```python
from build123d import *

# Parameters (mm, degrees)
SKETCH_2_W                 = 48
SKETCH_2_H                 = 75
EXTRUDE_1_DEPTH            = 10
EXTRUDE_2_DEPTH            = 55
EXTRUDE_2_DEPTH_BACK       = 10
SKETCH_5_W                 = 10
SKETCH_5_H                 = 10
EXTRUDE_2_2_DEPTH          = 55
EXTRUDE_2_2_DEPTH_BACK     = 10
SKETCH_5_H_2               = 20
EXTRUDE_2_3_DEPTH          = 55
EXTRUDE_2_3_DEPTH_BACK     = 10
EXTRUDE_2_4_DEPTH          = 55
EXTRUDE_2_4_DEPTH_BACK     = 10
EXTRUDE_3_DEPTH            = 5
SKETCH_7_R                 = 2.5
CUT_EXTRUDE_1_DEPTH        = 10
FILLET_1_R                 = 10
SKETCH_8_R                 = 1.5
CUT_EXTRUDE_2_DEPTH        = 121.205647632
PATTERN_LINEAR_1_COUNT     = 2
PATTERN_LINEAR_1_PITCH     = 15
PATTERN_LINEAR_1_COL_COUNT = 2
PATTERN_LINEAR_1_COL_PITCH = 15
SKETCH_10_R                = 1.5
CUT_EXTRUDE_4_DEPTH        = 10
SKETCH_11_R                = 1.5
CUT_EXTRUDE_5_DEPTH        = 5
FILLET_9_R                 = 2.5
EXTRUDE_5_DEPTH            = 5
FILLET_10_R                = 5
FILLET_11_R                = 5
SKETCH_14_R                = 1.5
CUT_EXTRUDE_6_DEPTH        = 5
SKETCH_15_W                = 5
SKETCH_15_H                = 2
CUT_EXTRUDE_7_DEPTH        = 55
SKETCH_17_R                = 1.5
CUT_EXTRUDE_10_DEPTH       = 118.336631714


with BuildPart() as part:
    # Sketch 2 → Extrude 1 (new body)
    with BuildSketch(Plane(origin=(0, 0, 0), x_dir=(0, 0, -1), z_dir=(1, 0, 0))):
        with Locations((22.061440678, -32.335805085)):
            Rectangle(SKETCH_2_W, SKETCH_2_H)
    extrude(amount=EXTRUDE_1_DEPTH)



with BuildPart() as body_2:
    # Sketch 5 → Extrude 2 (new, two sides: drawn at the far end of the back side and taken through both)
    with BuildSketch(Plane(origin=(10, 0, 0), x_dir=(0, 0, -1), z_dir=(1, 0, 0)).offset(-EXTRUDE_2_DEPTH_BACK)):
        with Locations((51.061440678, 0.164194915)):
            Rectangle(SKETCH_5_W, SKETCH_5_H)
    extrude(amount=EXTRUDE_2_DEPTH + EXTRUDE_2_DEPTH_BACK)


with BuildPart() as body_3:
    # Sketch 5 → Extrude 2 2 (new, two sides: drawn at the far end of the back side and taken through both)
    with BuildSketch(Plane(origin=(10, 0, 0), x_dir=(0, 0, -1), z_dir=(1, 0, 0)).offset(-EXTRUDE_2_2_DEPTH_BACK)):
        with Locations((51.061440678, -59.835805085)):
            Rectangle(SKETCH_5_W, SKETCH_5_H_2)
    extrude(amount=EXTRUDE_2_2_DEPTH + EXTRUDE_2_2_DEPTH_BACK)


with BuildPart() as body_4:
    # Sketch 5 → Extrude 2 3 (new, two sides: drawn at the far end of the back side and taken through both)
    with BuildSketch(Plane(origin=(10, 0, 0), x_dir=(0, 0, -1), z_dir=(1, 0, 0)).offset(-EXTRUDE_2_3_DEPTH_BACK)):
        with Locations((-6.938559322, -59.835805085)):
            Rectangle(SKETCH_5_W, SKETCH_5_H_2)
    extrude(amount=EXTRUDE_2_3_DEPTH + EXTRUDE_2_3_DEPTH_BACK)


with BuildPart() as body_5:
    # Sketch 5 → Extrude 2 4 (new, two sides: drawn at the far end of the back side and taken through both)
    with BuildSketch(Plane(origin=(10, 0, 0), x_dir=(0, 0, -1), z_dir=(1, 0, 0)).offset(-EXTRUDE_2_4_DEPTH_BACK)):
        with Locations((-6.938559322, 0.164194915)):
            Rectangle(SKETCH_5_W, SKETCH_5_H)
    extrude(amount=EXTRUDE_2_4_DEPTH + EXTRUDE_2_4_DEPTH_BACK)


with BuildPart() as part_1:
    add(part.part)

    add(body_3.part)  # Extrude 3 merges body 3

    add(body_4.part)  # Extrude 3 merges body 4
    # Sketch 6 → Extrude 3 (add)
    with BuildSketch(Plane.XZ.offset(69.835805085)):
        Polygon((65, 1.938559322), (65, 11.938559322), (0, 11.938559322), (0, 1.938559322), (0, -46.061440678), (0, -56.061440678), (65, -56.061440678), (65, -46.061440678), align=None)
    extrude(amount=EXTRUDE_3_DEPTH)

    # Sketch 7 → Cut-Extrude 1 (cut)
    with BuildSketch(Plane.ZY):
        with Locations((-22.061440678, -22.335805085)):
            Circle(SKETCH_7_R)
    extrude(amount=-CUT_EXTRUDE_1_DEPTH, mode=Mode.SUBTRACT)

    # Fillet 1
    fillet_1_edges = [part_1.edges().sort_by_distance(p)[0] for p in [
        (5, -49.835805085, -46.061440678),
        (5, -49.835805085, 1.938559322),
    ]]
    fillet(fillet_1_edges, radius=FILLET_1_R - 0.0001)  # a hair under: the kernel refuses the full size

    # Sketch 8 → Cut-Extrude 2 (cut, through all)
    with BuildSketch(Plane(origin=(0, 0, -56.061440678), x_dir=(-1, 0, 0), z_dir=(0, 0, -1))):
        with Locations((-32.5, -56.085805085)):
            Circle(SKETCH_8_R)
    cut_extrude_2 = extrude(amount=-CUT_EXTRUDE_2_DEPTH, mode=Mode.SUBTRACT)

    # Pattern Linear 1: Cut-Extrude 2 ×2
    with Locations(*[(i * PATTERN_LINEAR_1_PITCH, 0, 0) for i in range(1, PATTERN_LINEAR_1_COUNT)]):
        add(cut_extrude_2, mode=Mode.SUBTRACT)

    # Pattern Linear 1 col: Cut-Extrude 2 ×2
    with Locations(*[(-i * PATTERN_LINEAR_1_COL_PITCH, 0, 0) for i in range(1, PATTERN_LINEAR_1_COL_COUNT)]):
        add(cut_extrude_2, mode=Mode.SUBTRACT)

    # Sketch 10 → Cut-Extrude 4 (cut)
    with BuildSketch(Plane(origin=(0, -69.835805085, 0), x_dir=(1, 0, 0), z_dir=(0, 1, 0))):
        with Locations(Location((15, 2.632869249, 0), (0, 0, 270))):
            Circle(SKETCH_10_R)
        with Locations(Location((15, 41.490012107, 0), (0, 0, 270))):
            Circle(SKETCH_10_R)
    extrude(amount=-CUT_EXTRUDE_4_DEPTH, mode=Mode.SUBTRACT)

    # Sketch 11 → Cut-Extrude 5 (cut)
    with BuildSketch(Plane(origin=(65, 0, 0), x_dir=(0, 0, -1), z_dir=(1, 0, 0))):
        with Locations((51.061440678, -69.835805085)):
            Circle(SKETCH_11_R)
        with Locations((-6.938559322, -69.835805085)):
            Circle(SKETCH_11_R)
    extrude(amount=-CUT_EXTRUDE_5_DEPTH, mode=Mode.SUBTRACT)

    # Fillet 9
    fillet_9_edges = [part_1.edges().sort_by_distance(p)[0] for p in [
        (0, -62.335805085, -56.061440678),
        (0, -62.335805085, 11.938559322),
    ]]
    fillet(fillet_9_edges, radius=FILLET_9_R)


    add(body_2.part)  # Extrude 5 merges body 2

    add(body_5.part)  # Extrude 5 merges body 5
    # Sketch 13 → Extrude 5 (add)
    with BuildSketch(Plane(origin=(0, 5.164194915, 0), x_dir=(1, 0, 0), z_dir=(0, 1, 0))):
        Polygon((0, -11.938559322), (65, -11.938559322), (65, -1.938559322), (10, -1.938559322), (10, 46.061440678), (65, 46.061440678), (65, 56.061440678), (0, 56.061440678), (0, 46.061440678), (0, -1.938559322), align=None)
    extrude(amount=EXTRUDE_5_DEPTH)

    # Fillet 10
    fillet_10_edges = [part_1.edges().sort_by_distance(p)[0] for p in [
        (32.5, 10.164194915, 11.938559322),
        (32.5, -4.835805085, 11.938559322),
    ]]
    fillet(fillet_10_edges, radius=FILLET_10_R)

    # Fillet 11
    fillet_11_edges = [part_1.edges().sort_by_distance(p)[0] for p in [
        (32.5, 10.164194915, -56.061440678),
        (32.5, -4.835805085, -56.061440678),
    ]]
    fillet(fillet_11_edges, radius=FILLET_11_R)

    # Sketch 14 → Cut-Extrude 6 (cut)
    with BuildSketch(Plane(origin=(65, 0, 0), x_dir=(0, 0, -1), z_dir=(1, 0, 0))):
        with Locations((-6.938559322, 2.664194915)):
            Circle(SKETCH_14_R)
        with Locations((51.061440678, 2.664194915)):
            Circle(SKETCH_14_R)
    extrude(amount=-CUT_EXTRUDE_6_DEPTH, mode=Mode.SUBTRACT)

    # Sketch 15 → Cut-Extrude 7 (cut)
    with BuildSketch(Plane(origin=(65, 0, 0), x_dir=(0, 0, -1), z_dir=(1, 0, 0))):
        with Locations((22.061440678, -70.835805085)):
            Rectangle(SKETCH_15_W, SKETCH_15_H)
    extrude(amount=-CUT_EXTRUDE_7_DEPTH, mode=Mode.SUBTRACT)

    # Sketch 17 → Cut-Extrude 10 (cut, through all)
    with BuildSketch(Plane(origin=(0, -69.835805085, 0), x_dir=(1, 0, 0), z_dir=(0, 1, 0))):
        with Locations(Location((60.5, 22.061440678, 0), (0, 0, 270))):
            Circle(SKETCH_17_R)
        with Locations(Location((46.5, 22.061440678, 0), (0, 0, 270))):
            Circle(SKETCH_17_R)
        with Locations(Location((53.5, 29.061440678, 0), (0, 0, 270))):
            Circle(SKETCH_17_R)
        with Locations(Location((53.5, 22.061440678, 0), (0, 0, 270))):
            Circle(SKETCH_17_R)
        with Locations(Location((53.5, 15.061440678, 0), (0, 0, 270))):
            Circle(SKETCH_17_R)
        with Locations(Location((32.5, 15.061440678, 0), (0, 0, 270))):
            Circle(SKETCH_17_R)
        with Locations(Location((39.5, 22.061440678, 0), (0, 0, 270))):
            Circle(SKETCH_17_R)
        with Locations(Location((25.5, 22.061440678, 0), (0, 0, 270))):
            Circle(SKETCH_17_R)
        with Locations(Location((32.5, 22.061440678, 0), (0, 0, 270))):
            Circle(SKETCH_17_R)
        with Locations(Location((32.5, 29.061440678, 0), (0, 0, 270))):
            Circle(SKETCH_17_R)
    extrude(amount=-CUT_EXTRUDE_10_DEPTH, mode=Mode.SUBTRACT)


solid = part_1.part
```
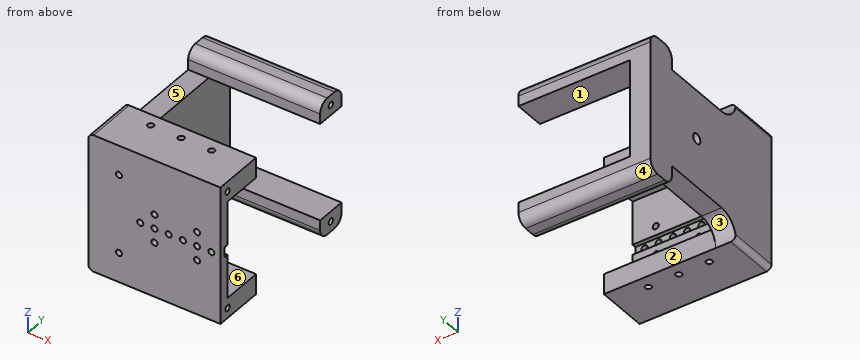
Input: part model. Units: mm. Frame: model coordinates. Face numbers are marked on the shaded views. A direction names the side the tool comes from. Give positions to 0.01 mm unless a question says otherwise; leave off trailing zeros. Order: outer loops, then holes, each group sorted by start corner. A loop starts at its lowest first (then second) coordinate and runs counter-clockwise, first axis right, second up. Notation, with made-up numbers: (36.25, 62) -> (55.25, 62) arc R27 ccw to (55.25, 79) -> close; hole circle Ø3 at (-13.75, 76.5). An arc over 180 degrees is marked (long way). Write each question's results on one line, items separated by ' | '. Start each with the question number.
Item 1: Set-up query: the marked faces 1, 2 and 3. Return all of +Z, -Z, +X, -X, +Y, -Y with unobstructed straight access to the full face (end or side cutting, diameter ignored); none if empty.
Item 2: Cut plane A-A on x = 25.5. Return the cut outline in (y, z).
Item 3: Cut plane C-C on x = 36. Return the cut outline in (y, z), then the cut area to 3 significant figures.
Item 4: Line query: line 1 (Y direction, x = 47.5, z = 4); line 2 (Y direction, x = 29, z = -48); line 3 (Z direction, x = 21, y = -63). Output: solid intervals per line, ascending.
Item 5: Cut plane D-D on z = -22. Give the number of separate pieces and of enclosed holes in the cut face, then the cut area to 3 significant figures.
Item 6: Mould query, pull axis Z, two halves, no side actions, for the marked faces 4, 5 and 6. Classes: pulls with the +Z half, pulls with the -Z half, needs draft (parallel to the pull), parting line crosses it, or undercut.
Item 7: Cut plane B-B on z = -15. Return the cut outline in (x, y).
Item 8: Contact query for flat-ended pins moving along their axis: P1, Ø5, axis at x = 55, y = -4, coming from the +Z side; P2, Ø8, axis at y = -36.5, z = -45.5, coming from the +X side; P3, Ø6, axis at x = 48.5, z = -17, coming from the +Y side. Output: stop coordinate, or through.
Established:
1) face 1: +X, +Y | face 2: +Z, -Z, +X | face 3: -Z, +X, -X
2) outline: (-74.84, -56.06) -> (-49.84, -56.06) -> (-49.84, -46.06) -> (-69.84, -46.06) -> (-69.84, -24.56) -> (-71.84, -24.56) -> (-71.84, -23.56) -> (-74.84, -23.56) -> close; (-74.84, -20.56) -> (-71.84, -20.56) -> (-71.84, -19.56) -> (-69.84, -19.56) -> (-69.84, 1.94) -> (-49.84, 1.94) -> (-49.84, 11.94) -> (-74.84, 11.94) -> close; (-4.84, -51.06) arc R5 ccw to (0.16, -56.06) -> (5.16, -56.06) arc R5 ccw to (10.16, -51.06) -> (10.16, -46.06) -> (-4.84, -46.06) -> close; (-4.84, 1.94) -> (10.16, 1.94) -> (10.16, 6.94) arc R5 ccw to (5.16, 11.94) -> (0.16, 11.94) arc R5 ccw to (-4.84, 6.94) -> close
3) outline: (-74.84, -56.06) -> (-49.84, -56.06) -> (-49.84, -46.06) -> (-69.84, -46.06) -> (-69.84, -24.56) -> (-71.84, -24.56) -> (-71.84, -19.56) -> (-69.84, -19.56) -> (-69.84, 1.94) -> (-49.84, 1.94) -> (-49.84, 11.94) -> (-74.84, 11.94) -> close; (-4.84, -51.06) arc R5 ccw to (0.16, -56.06) -> (5.16, -56.06) arc R5 ccw to (10.16, -51.06) -> (10.16, -46.06) -> (-4.84, -46.06) -> close; (-4.84, 1.94) -> (10.16, 1.94) -> (10.16, 6.94) arc R5 ccw to (5.16, 11.94) -> (0.16, 11.94) arc R5 ccw to (-4.84, 6.94) -> close | area: 1,010 mm^2
4) line 1: -74.84 to -57.59, -54.59 to -49.84, -4.84 to 10.16 | line 2: -74.84 to -49.84, -4.84 to 10.16 | line 3: -56.06 to -46.06, 1.94 to 11.94
5) separate pieces: 8 | enclosed holes: 0 | area: 911 mm^2
6) face 4: pulls with the -Z half | face 5: pulls with the +Z half | face 6: undercut
7) outline: (0, -74.84) -> (31, -74.84) -> (31, -69.84) -> (10, -69.84) -> (10, 10.16) -> (0, 10.16) -> close; (34, -74.84) -> (52, -74.84) -> (52, -69.84) -> (34, -69.84) -> close; (55, -74.84) -> (65, -74.84) -> (65, -69.84) -> (55, -69.84) -> close
8) P1: z = 11.65 | P2: x = 10 | P3: y = -69.84
